from build123d import *

# Parameters (mm, degrees)
F1_DEPTH = 34
F2_R     = 1.1
F4_DEPTH = 1.2
F5_R     = 3


with BuildPart() as f1:
    # F0 (on Top) → F1 (new body, symmetric)
    with BuildSketch(Plane.XY):
        with BuildLine():
            Line((17.2, 1.6774998092), (17.2, 3.4427671539))
            ThreePointArc((17.2, 3.4427671539), (0, 10.3), (-17.2, 3.4427671539))
            Line((-17.2, 3.4427671539), (-17.2, 1.6774998092))
            ThreePointArc((-17.2, 1.6774998092), (0, 9.05), (17.2, 1.6774998092))
        make_face()
    extrude(amount=F1_DEPTH, both=True)

    # F2 (on Front) → F3 (join, up to the next surface of F1)
    with BuildSketch(Plane.XZ):
        with BuildLine():
            Line((15.3, 29.1), (17.2, 29.1))
            Line((17.2, 29.1), (17.2, 34))
            Line((17.2, 34), (12.3, 34))
            Line((12.3, 34), (12.3, 32.1))
            ThreePointArc((12.3, 32.1), (13.1786796564, 29.9786796564), (15.3, 29.1))
        make_face()
        with Locations((14.75, 31.55)):
            Circle(F2_R, mode=Mode.SUBTRACT)
        with BuildLine():
            Line((-12.3, 34), (-17.2, 34))
            Line((-17.2, 34), (-17.2, 29.1))
            Line((-17.2, 29.1), (-15.3, 29.1))
            ThreePointArc((-15.3, 29.1), (-13.1786796564, 29.9786796564), (-12.3, 32.1))
            Line((-12.3, 32.1), (-12.3, 34))
        make_face()
        with Locations((-14.75, 31.55)):
            Circle(F2_R, mode=Mode.SUBTRACT)
        with Locations((14.75, 31.55)):
            Circle(F2_R)
        with Locations((-14.75, 31.55)):
            Circle(F2_R)
        with BuildLine():
            Line((-15.3, -29.1), (-17.2, -29.1))
            Line((-17.2, -29.1), (-17.2, -34))
            Line((-17.2, -34), (-12.3, -34))
            Line((-12.3, -34), (-12.3, -32.1))
            ThreePointArc((-12.3, -32.1), (-13.1786796564, -29.9786796564), (-15.3, -29.1))
        make_face()
        with Locations((-14.75, -31.55)):
            Circle(F2_R, mode=Mode.SUBTRACT)
        with Locations((-14.75, -31.55)):
            Circle(F2_R)
        with BuildLine():
            Line((12.3, -34), (17.2, -34))
            Line((17.2, -34), (17.2, -29.1))
            Line((17.2, -29.1), (15.3, -29.1))
            ThreePointArc((15.3, -29.1), (13.1786796564, -29.9786796564), (12.3, -32.1))
            Line((12.3, -32.1), (12.3, -34))
        make_face()
        with Locations((14.75, -31.55)):
            Circle(F2_R, mode=Mode.SUBTRACT)
        with Locations((14.75, -31.55)):
            Circle(F2_R)
    extrude(until=Until.NEXT, dir=(0, 1, 0))

    # F2 (on Front) → F4 (cut)
    with BuildSketch(Plane.XZ):
        with Locations((-14.75, -31.55)):
            Circle(F2_R)
        with Locations((-14.75, 31.55)):
            Circle(F2_R)
        with Locations((14.75, 31.55)):
            Circle(F2_R)
        with Locations((14.75, -31.55)):
            Circle(F2_R)
    extrude(amount=-F4_DEPTH, mode=Mode.SUBTRACT)

    # F5
    f5_edges = [f1.edges().sort_by_distance(p)[0] for p in [
        (-17.2, 1.721384, 34),
        (17.2, 1.721384, 34),
        (-17.2, 1.721384, -34),
        (17.2, 1.721384, -34),
    ]]
    fillet(f5_edges, radius=F5_R)


solid = f1.part
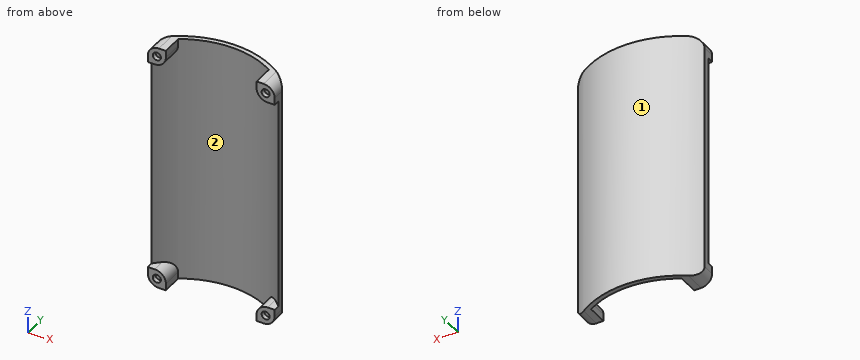
Could you check a few things on this model? Use its own coordinates, in mm. Face numbers are marked on the shaded views. Coordinates: 2 decimals unless noted, no trailing zeros. Order: outer loops, then holes, each group sorted by start corner. A loop starts at its lowest first (then second) coordinate and runs counter-clockwise, first axis right, second up.
Q1. Suppose I cut it at D-D on y = 4.25. Please give me the cut outline in (x, z), and give its area (3 significant figures).
Q2. Suppose I cut it at A-A on y = 8.25. Please give me the cut outline in (x, z).
Q3. Please list where these lines run through material, in increasing order: L1, parallel to Z at x = 14.75, y = 0.25; L2, parallel to X at y = 6.25, z = 1; L3, parallel to X at y = 5.75, z = 26.5.
Q4. Thinking about a two-plate mould opening in Z: for the marked faces 1 and 2, which applies, released by +Z, released by -Z, zero draft, split by the parting line, or undercut?
Q5. Suppose I cut it at B-B on x = -6. Please give me the cut outline in (y, z).
Q6. Will these pins go through, and if not, where does the flat tip stop? pin 1 (2.5 mm diameter, centred on x = -14.75, z = 31.55, fed in from -Y); pin 2 (1.5 mm diameter, centred on y = 1.5, z = -33.5, fed in from +X); pin 3 (1 mm diameter, centred on x = 6, z = 21, fed in from +Y); pin 4 (1.5 mm diameter, centred on y = 4.5, z = -14.5, fed in from +X).
Q7. Suppose I cut it at C-C on z = 8. Please give me the cut outline in (x, y).
Answer:
1. outline: (-16.31, -33.14) arc R3 ccw to (-14.2, -34) - (-12.3, -34) - (-12.3, -32.1) arc R3 ccw to (-14.32, -29.27) - (-14.32, 29.27) arc R3 ccw to (-12.3, 32.1) - (-12.3, 34) - (-14.2, 34) arc R3 ccw to (-16.31, 33.14) - close; (12.3, -34) - (14.2, -34) arc R3 ccw to (16.31, -33.14) - (16.31, 33.14) arc R3 ccw to (14.2, 34) - (12.3, 34) - (12.3, 32.1) arc R3 ccw to (14.32, 29.27) - (14.32, -29.27) arc R3 ccw to (12.3, -32.1) - close
1. area: 300 mm2
2. outline: (-9.91, -34) - (-6.11, -34) - (-6.11, 34) - (-9.91, 34) - close; (6.11, -34) - (9.91, -34) - (9.91, 34) - (6.11, 34) - close
3. L1: z = -33.95 to -32.65, -30.45 to -29.15, 29.15 to 30.45, 32.65 to 33.95
3. L2: x = -13.64 to -11.19, 11.19 to 13.64
3. L3: x = -14.38 to -12.08, 12.08 to 14.38
4. face 1: zero draft
4. face 2: undercut
5. outline: (8.28, -34) - (9.57, -34) - (9.57, 34) - (8.28, 34) - close
6. pin 1: stops at y = 0
6. pin 2: stops at x = 16.64
6. pin 3: stops at y = 9.69
6. pin 4: stops at x = 16.87
7. outline: (-17.2, 1.68) arc R23.75 cw to (17.2, 1.68) - (17.2, 3.44) arc R25 ccw to (-17.2, 3.44) - close
